Design review of the part shown in the three views and the two pictorial views. Dimensions are in mm from the part's minimum x, y and z. Coordinates: 2 decimals unless noted, no trailing zeros. Loops run counter-clockwise (first coordinate to the right, second up) from the corner with the lowest first, then second, coordinate; pieces in that order, holes last. Notation, with made-up numbers: (-32, -16) -> (26, -16) arc R28 ccw to (26, 5) -> close; hole circle Ø7 at (47.5, 19). An arc over 180 degrees is marked (long way). One line per item, written item: value. Start each with the question number.
1. Insertion check: pin 1 (2.5 mm diameter, centred on x = 81.5, z = 7.5, fed in from -Y); pin 2 (13.5 mm diameter, centred on x = 64, y = 31.5, fed in from +Z); pin 3 (2.5 mm diameter, centred on x = 64.5, y = 41, fed in from +Z). Each pin has a flat end and moves straight along its axis. Give the tip position at first contact, or say it passes through.
2. Add section C-C on y = 22.5. Write out the cut boundary in (x, z).
3. For probe 1 along X at (y, z) = (39, 2.5) (1 decimal); probe 2 along X at (y, z) = (21, 7) (1 decimal); probe 3 along X at (y, z) = (23, 3.25), list the stretches that pass through material, from the lowest coordinate up.
4. Add section A-A on z = 7.75. Write out the cut boundary in (x, y).
5. Add section B-B on x = 7.5. Write out the cut boundary in (y, z).
6. Add section D-D on z = 4. Write out the cut boundary in (x, y).
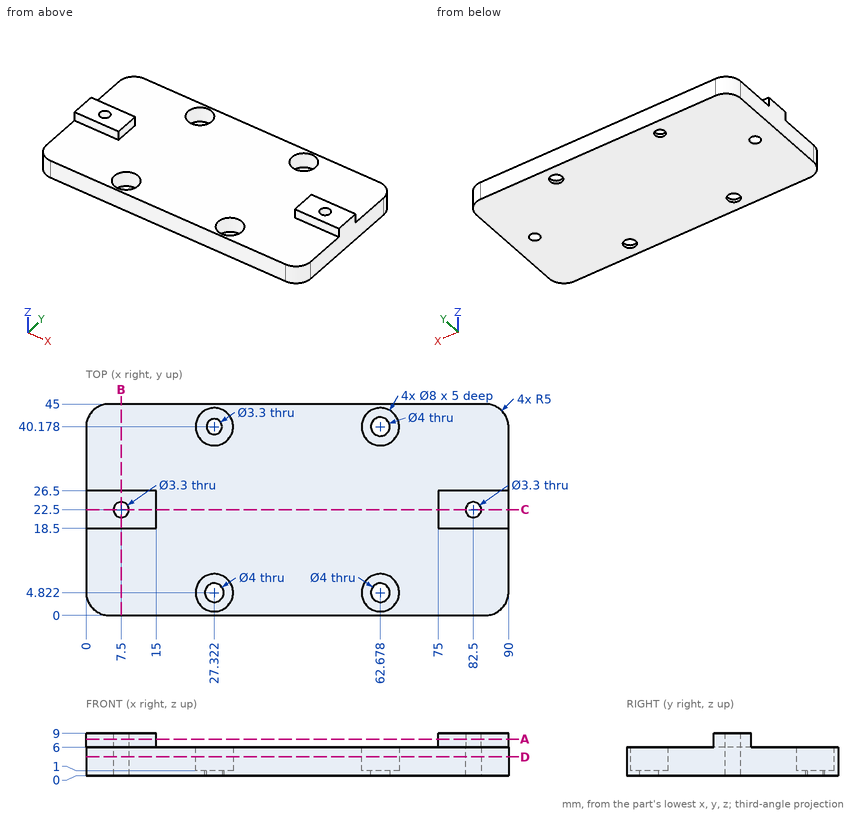
Worked answers:
1. pin 1: stops at y = 18.5
1. pin 2: stops at z = 6
1. pin 3: stops at z = 1
2. outline: (0, 0) -> (5.85, 0) -> (5.85, 9) -> (0, 9) -> close; (9.15, 0) -> (80.85, 0) -> (80.85, 9) -> (75, 9) -> (75, 6) -> (15, 6) -> (15, 9) -> (9.15, 9) -> close; (84.15, 0) -> (90, 0) -> (90, 9) -> (84.15, 9) -> close
3. probe 1: x = 0 to 23.5, 31.1 to 58.9, 66.5 to 90
3. probe 2: x = 0 to 6.8, 8.2 to 15, 75 to 81.8, 83.2 to 90
3. probe 3: x = 0 to 5.93, 9.07 to 80.93, 84.07 to 90
4. outline: (0, 18.5) -> (15, 18.5) -> (15, 26.5) -> (0, 26.5) -> close; (75, 18.5) -> (90, 18.5) -> (90, 26.5) -> (75, 26.5) -> close; hole circle Ø3.3 at (7.5, 22.5); hole circle Ø3.3 at (82.5, 22.5)
5. outline: (0, 0) -> (20.85, 0) -> (20.85, 9) -> (18.5, 9) -> (18.5, 6) -> (0, 6) -> close; (24.15, 0) -> (45, 0) -> (45, 6) -> (26.5, 6) -> (26.5, 9) -> (24.15, 9) -> close
6. outline: (0, 5) arc R5 ccw to (5, 0) -> (85, 0) arc R5 ccw to (90, 5) -> (90, 40) arc R5 ccw to (85, 45) -> (5, 45) arc R5 ccw to (0, 40) -> close; hole circle Ø3.3 at (7.5, 22.5); hole circle Ø8 at (27.32, 4.82); hole circle Ø8 at (27.32, 40.18); hole circle Ø8 at (62.68, 4.82); hole circle Ø8 at (62.68, 40.18); hole circle Ø3.3 at (82.5, 22.5)
